The listing builds one solid part. Answer for the finished solid, in the listing's coordinates (mm). Face numbers are marked on the shaded views. A direction names the side the tool comes from. Round coordinates to 2 decimals unless told otherwise and drop trailing zeros. Loops run counter-clockwise (first coordinate to the right, second up) from the corner with the lowest first, then second, coordinate; pieces in that order, holes last. Notation, with made-up numbers: M 46.5,0 L 91.5,0 A25 cw 91.5,13 Z; hole C 27.25,-20 d5. An arc over 180 degrees is marked long. Put each result on its own line as item: value. Start each with the question number.
(1) Straight lines are drawn through the part: line 1 (Z direction, x = 13, y = 67); line 2 (X direction, y = 37.5, z = -26.5); line 3 (Y direction, x = 103, z = -33). For each, find the intervals that lie inside material, in ascending order.
(2) Which of the six approach directions +Z, -Z, +X, -X, +Y, -Y give full straight-line access (tool end or side, diameter ignored) to the marked faces 1, 2, 3, 4 and 5?
(3) Section D-D, the plane x = 136 is taken. Determine the outline of the cut face in (y, z), then the cut area to 3 significant figures.
(4) Section B-B, the plane x = 99 is taken. Determine the outline of the cut face in (y, z).
(5) Flat-ended cylindrical pins translate along their axes: P1, Ø6, axis at y = 110, z = -80, coming from the -X side; P2, Ø0.6, axis at y = 9, z = -97.5, coming from the +X side; P3, Ø3, axis at x = 112, z = -50, coming from the -Y side. Find the tip coordinate at first contact, or state that the pin passes through.
(6) Determine the mould class of the marked faces 6, 7 and 8 for opening direction Z: released by +Z, released by -Z, zero draft, split by the parting line, or undercut.
(7) Section C-C, the plane z = -88.5 is taken. Determine the outline of the cut face in (x, y), then the cut area to 3 significant figures.
(8) Section A-A, the plane y = 15 is taken. Determine the outline of the cut face in (x, z).
```python
from build123d import *

# Parameters (mm, degrees)
ESBO_O1_W                   = 110
ESBO_O1_H                   = 160
RESSALTO_EXTRUS_O1_DEPTH    = 10
ESBO_O2_W                   = 95
ESBO_O2_H                   = 140
CORTE_EXTRUS_O1_DEPTH       = 2
RESSALTO_EXTRUS_O2_DEPTH    = 110
ESBO_O6_W                   = 25.003576957
ESBO_O6_H                   = 20
CORTE_EXTRUS_O2_DEPTH       = 10
ESBO_O7_W                   = 140
ESBO_O7_H                   = 20.035722947
SAIDAPRAFIOSSENSORES_DEPTH  = 30
ESBO_O8_W                   = 140
ESBO_O8_H                   = 9.973523328
SUPORTE_PARA_SENSORES_DEPTH = 55
ESBO_O9_W                   = 55
ESBO_O9_H                   = 140
CORTE_EXTRUS_O4_DEPTH       = 2
ESBO_O5_W                   = 110
ESBO_O5_H                   = 160
RESSALTO_EXTRUS_O3_DEPTH    = 10
ESBO_O11_W                  = 5
ESBO_O11_H                  = 21
CORTE_EXTRUS_O5_DEPTH       = 9
ESBO_O12_W                  = 102.5
ESBO_O12_H                  = 140
CORTE_EXTRUS_O6_DEPTH       = 7
CORTE_EXTRUS_O7_DEPTH       = 7
CORTE_EXTRUS_O8_DEPTH       = 7
ESBO_O15_W                  = 110
ESBO_O15_H                  = 160
CORTE_EXTRUS_O9_DEPTH       = 5
ESBO_O16_W                  = 154
ESBO_O16_H                  = 119
CORTE_EXTRUS_O10_DEPTH      = 4.5
ESBO_O17_W                  = 55
ESBO_O17_H                  = 140
CORTE_EXTRUS_O11_DEPTH      = 5
ESBO_O18_W                  = 55
ESBO_O18_H                  = 2.973523328
RESSALTO_EXTRUS_O4_DEPTH    = 7
ESBO_O19_W                  = 55
ESBO_O19_H                  = 2.973523328
RESSALTO_EXTRUS_O5_DEPTH    = 7
RESSALTO_EXTRUS_O6_DEPTH    = 2


with BuildPart() as part:
    # Esboço1 → Ressalto-extrusão1 (new body)
    with BuildSketch(Plane(origin=(0, 0, 0), x_dir=(1, 0, 0), z_dir=(0, 1, 0))):
        with Locations((55, 80)):
            Rectangle(ESBO_O1_W, ESBO_O1_H)
    extrude(amount=RESSALTO_EXTRUS_O1_DEPTH)

    # Esboço2 → Corte-extrusão1 (cut)
    with BuildSketch(Plane(origin=(0, 10, 0), x_dir=(1, 0, 0), z_dir=(0, 1, 0))):
        with Locations((55, 80)):
            Rectangle(ESBO_O2_W, ESBO_O2_H)
    extrude(amount=-CORTE_EXTRUS_O1_DEPTH, mode=Mode.SUBTRACT)

    # Esboço4 → Ressalto-extrusão2 (add)
    with BuildSketch(Plane(origin=(0, 10, 0), x_dir=(1, 0, 0), z_dir=(0, 1, 0))):
        Polygon((0, 160), (0, 150), (102.5, 150), (102.5, 10), (0, 10), (0, 0), (110, 0), (110, 160), align=None)
    extrude(amount=RESSALTO_EXTRUS_O2_DEPTH)

    # Esboço6 → Corte-extrusão2 (cut)
    with BuildSketch(Plane.XY.offset(-150)):
        with Locations((45.020695382, 18)):
            Rectangle(ESBO_O6_W, ESBO_O6_H)
    extrude(amount=-CORTE_EXTRUS_O2_DEPTH, mode=Mode.SUBTRACT)

    # Esboço7 → Saidaprafiossensores (cut)
    with BuildSketch(Plane.ZY.offset(-102.5)):
        with Locations((-80, 48.022769051)):
            Rectangle(ESBO_O7_W, ESBO_O7_H)
    extrude(amount=-SAIDAPRAFIOSSENSORES_DEPTH, mode=Mode.SUBTRACT)

    # Esboço8 → Suporte para sensores (add)
    with BuildSketch(Plane(origin=(110, 0, 0), x_dir=(0, 0, -1), z_dir=(1, 0, 0))):
        with Locations((80, 33.018145913)):
            Rectangle(ESBO_O8_W, ESBO_O8_H)
    extrude(amount=SUPORTE_PARA_SENSORES_DEPTH)

    # Esboço9 → Corte-extrusão4 (cut)
    with BuildSketch(Plane(origin=(0, 38.004907577, 0), x_dir=(1, 0, 0), z_dir=(0, 1, 0))):
        with Locations((137.5, 80)):
            Rectangle(ESBO_O9_W, ESBO_O9_H)
    extrude(amount=-CORTE_EXTRUS_O4_DEPTH, mode=Mode.SUBTRACT)

    # Esboço5 → Ressalto-extrusão3 (add)
    with BuildSketch(Plane(origin=(0, 120, 0), x_dir=(1, 0, 0), z_dir=(0, 1, 0))):
        with Locations((55, 80)):
            Rectangle(ESBO_O5_W, ESBO_O5_H)
    extrude(amount=RESSALTO_EXTRUS_O3_DEPTH)

    # Esboço11 → Corte-extrusão5 (cut)
    with BuildSketch(Plane(origin=(0, 130, 0), x_dir=(1, 0, 0), z_dir=(0, 1, 0))):
        with Locations((82.5, 74.263561318)):
            Rectangle(ESBO_O11_W, ESBO_O11_H)
    extrude(amount=-CORTE_EXTRUS_O5_DEPTH, mode=Mode.SUBTRACT)

    # Esboço12 → Corte-extrusão6 (cut)
    with BuildSketch(Plane.XZ.offset(-120)):
        with Locations((51.25, -80)):
            Rectangle(ESBO_O12_W, ESBO_O12_H)
    extrude(amount=-CORTE_EXTRUS_O6_DEPTH, mode=Mode.SUBTRACT)

    # Esboço13 → Corte-extrusão7 (cut)
    with BuildSketch(Plane.XY.offset(-150)):
        Polygon((7.5, 8), (7.5, 10), (0, 10), (0, 127), (102.5, 127), (102.5, 58.040630524), (110, 58.040630524), (110, 38.004907577), (102.5, 38.004907577), (102.5, 8), align=None)
    extrude(amount=-CORTE_EXTRUS_O7_DEPTH, mode=Mode.SUBTRACT)

    # Esboço14 → Corte-extrusão8 (cut)
    with BuildSketch(Plane(origin=(0, 0, -10), x_dir=(-1, 0, 0), z_dir=(0, 0, -1))):
        Polygon((-102.5, 127), (0, 127), (0, 10), (-7.5, 10), (-7.5, 8), (-102.5, 8), (-102.5, 38.004907577), (-110, 38.004907577), (-110, 58.040630524), (-102.5, 58.040630524), align=None)
    extrude(amount=-CORTE_EXTRUS_O8_DEPTH, mode=Mode.SUBTRACT)

    # Esboço15 → Corte-extrusão9 (cut)
    with BuildSketch(Plane.XZ):
        with Locations((55, -80)):
            Rectangle(ESBO_O15_W, ESBO_O15_H)
    extrude(amount=-CORTE_EXTRUS_O9_DEPTH, mode=Mode.SUBTRACT)

    # Esboço16 → Corte-extrusão10 (cut)
    with BuildSketch(Plane.ZY.offset(-102.5)):
        with Locations((-80, 67.5)):
            Rectangle(ESBO_O16_W, ESBO_O16_H)
    extrude(amount=-CORTE_EXTRUS_O10_DEPTH, mode=Mode.SUBTRACT)

    # Esboço17 → Corte-extrusão11 (cut)
    with BuildSketch(Plane.XZ.offset(-28.031384249)):
        with Locations((137.5, -80)):
            Rectangle(ESBO_O17_W, ESBO_O17_H)
    extrude(amount=-CORTE_EXTRUS_O11_DEPTH, mode=Mode.SUBTRACT)

    # Esboço18 → Ressalto-extrusão4 (add)
    with BuildSketch(Plane.XY.offset(-10)):
        with Locations((137.5, 34.518145913)):
            Rectangle(ESBO_O18_W, ESBO_O18_H)
    extrude(amount=RESSALTO_EXTRUS_O4_DEPTH)

    # Esboço19 → Ressalto-extrusão5 (add)
    with BuildSketch(Plane(origin=(0, 0, -150), x_dir=(-1, 0, 0), z_dir=(0, 0, -1))):
        with Locations((-137.5, 34.518145913)):
            Rectangle(ESBO_O19_W, ESBO_O19_H)
    extrude(amount=RESSALTO_EXTRUS_O5_DEPTH)

    # Esboço20 → Ressalto-extrusão6 (add)
    with BuildSketch(Plane(origin=(0, 36.004907577, 0), x_dir=(1, 0, 0), z_dir=(0, 1, 0))):
        Polygon((110, 157), (110, 156.007066328), (164.030852529, 156.007066328), (164.030852529, 4.050019812), (110, 4.050019812), (110, 3), (165, 3), (165, 157), align=None)
    extrude(amount=RESSALTO_EXTRUS_O6_DEPTH)


solid = part.part
```
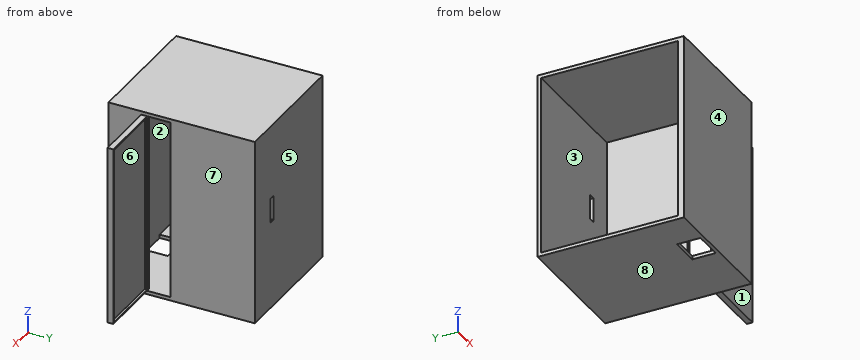
Recorded:
1. line 1: z = -160 to -157, -3 to 0
1. line 2: x = 107 to 110, 164.03 to 165
1. line 3: y = 5 to 8, 127 to 130
2. face 1: +Z, -Z, +X, -Y
2. face 2: none
2. face 3: -X
2. face 4: +Z, -Z, +X, -X, -Y
2. face 5: +Z, -Z, +X, -X, +Y
3. outline: M 33.03,-157 L 38,-157 L 38,-156.01 L 36,-156.01 L 36,-4.05 L 38,-4.05 L 38,-3 L 33.03,-3 Z
3. area: 462 mm²
4. outline: M 5,-160 L 130,-160 L 130,0 L 5,0 Z; hole M 8,-157 L 127,-157 L 127,-3 L 8,-3 Z
5. P1: stops at x = 107
5. P2: stops at x = 110
5. P3: stops at y = 33.03
6. face 6: undercut
6. face 7: zero draft
6. face 8: released by -Z
7. outline: M 0,5 L 110,5 L 110,33.03 L 165,33.03 L 165,38 L 164.03,38 L 164.03,36 L 110,36 L 110,38 L 107,38 L 107,8 L 7.5,8 L 7.5,10 L 0,10 Z; M 0,127 L 107,127 L 107,58.04 L 110,58.04 L 110,130 L 0,130 Z
7. area: 1,140 mm²
8. outline: M 0,-160 L 32.52,-160 L 32.52,-157 L 0,-157 Z; M 0,-3 L 107,-3 L 107,-157 L 57.52,-157 L 57.52,-160 L 110,-160 L 110,0 L 0,0 Z
